from build123d import *

# Parameters (mm, degrees)
BOSS_EXTRUDE1_START = -3.18
SKETCH1_W           = 16.037750947
SKETCH1_H           = 13.801978015
BOSS_EXTRUDE1_DEPTH = 3.18
SKETCH3_W           = 15.364094043
SKETCH3_H           = 13.801978015
SKETCH3_R           = 2.5
BOSS_EXTRUDE2_DEPTH = 3.18


with BuildPart() as part:
    # Sketch1 → Boss-Extrude1 (new body)
    with BuildSketch(Plane.XY.offset(BOSS_EXTRUDE1_START)):
        with Locations((15.890651203, -26.571727946)):
            Rectangle(SKETCH1_W, SKETCH1_H)
    extrude(amount=-BOSS_EXTRUDE1_DEPTH)

    # Sketch3 → Boss-Extrude2 (add)
    with BuildSketch(Plane.ZY.offset(-7.871775729)):
        with Locations((1.322047021, -26.571727946)):
            Rectangle(SKETCH3_W, SKETCH3_H)
        with Locations(Location((4.053672899, -26.571727946, 0), (0, 0, 180))):
            Circle(SKETCH3_R, mode=Mode.SUBTRACT)
    extrude(amount=BOSS_EXTRUDE2_DEPTH)


solid = part.part
Check sheet for the modelled part. Datum: model origin and axes. Units: mm. A direction names the side the tool comes from. Coordinates: 2 decimals unless noted, no trailing zeros. Loops run counter-clockwise (first coordinate to the right, second up) from the corner with the lowest first, then second, coordinate; pieces in that order, holes last. Notation, with made-up numbers: (-31.5, 47) -> (-21.5, 47) arc R18 cw to (-21.5, 70) -> close; hole circle Ø10 at (65.25, 51.25). An arc over 180 degrees is marked (long way). Answer in a Markdown table with one row per item.
1. Sectioned sample at B-B, the plane y = -27.25. Record the boundary of the cut face in (x, z).
Check values:
| item | result |
|---|---|
| outline | (4.69, -6.36) -> (23.91, -6.36) -> (23.91, -3.18) -> (7.87, -3.18) -> (7.87, 1.65) -> (4.69, 1.65) -> close; (4.69, 6.46) -> (7.87, 6.46) -> (7.87, 9) -> (4.69, 9) -> close |
2. Sectioned sample at C-C, the plane x = 19.25. Record the boundary of the cut face in (y, z), then the cut area to 3 significant figures.
Check values:
| item | result |
|---|---|
| outline | (-33.47, -6.36) -> (-19.67, -6.36) -> (-19.67, -3.18) -> (-33.47, -3.18) -> close |
| area | 43.9 mm2 |
3. Release check for a two-part mould opening along Z. For faces 3 (the face through (12, -19.671, -4)), 4 (the face through (6.3, -26.68, 6.55)), 5 (the face through (14, -27, -6.36)) record: released by +Z, released by -Z, zero draft, split by the parting line, or undercut.
Check values:
| item | result |
|---|---|
| face 3 | zero draft |
| face 4 | undercut |
| face 5 | released by -Z |
4. Material ranges on line 1 along Z through (x, y) = (12.5, -31.5); line 2 along X through (y, z) = (-31.25, 1.5); line 3 along Z through (x, y) = (7.5, -25.75), recorded low to high. Write a range as [from, to].
Check values:
| item | result |
|---|---|
| line 1 | z = [-6.36, -3.18] |
| line 2 | x = [4.69, 7.87] |
| line 3 | z = [-6.36, 1.69], [6.41, 9] |
5. Go/stop test with flat-tipped pins: pin 1 (6.5 mm diameter, centred on y = -26.57, z = 4.05, fed in from +X); pin 2 (4 mm diameter, centred on x = 13.5, y = -24, fed in from +Z). Record where each tip stops, or that it passes through.
Check values:
| item | result |
|---|---|
| pin 1 | stops at x = 7.87 |
| pin 2 | stops at z = -3.18 |
6. Sectioned sample at D-D, the plane z = 7. Record the boundary of the cut face in (x, y), then the cut area to 3 significant figures.
Check values:
| item | result |
|---|---|
| outline | (4.69, -33.47) -> (7.87, -33.47) -> (7.87, -19.67) -> (4.69, -19.67) -> close |
| area | 43.9 mm2 |
7. Access from +Z, -Z, +X, -X, +Y, -Y to the whole of each face (thin tool, end or side, straight path). Record for faces 1 (the face through (4.692, -26, 1)), 2 (the face through (7.872, -26, 1)).
Check values:
| item | result |
|---|---|
| face 1 | +Z, -Z, -X, +Y, -Y |
| face 2 | +Z, +X, +Y, -Y |
8. Sectioned sample at A-A, the plane z = 4.5. Record the boundary of the cut face in (x, y), then the cut area to 3 significant figures.
Check values:
| item | result |
|---|---|
| outline | (4.69, -33.47) -> (7.87, -33.47) -> (7.87, -29.03) -> (4.69, -29.03) -> close; (4.69, -24.11) -> (7.87, -24.11) -> (7.87, -19.67) -> (4.69, -19.67) -> close |
| area | 28.2 mm2 |
